```python
from build123d import *

# Parameters (mm, degrees)
F0_R     = 14.534071
F1_DEPTH = 4
F2_R     = 9.020601
F3_DEPTH = 55.9
F4_R     = 12.826106
F4_R_2   = 10.112728
F5_DEPTH = 67.3


with BuildPart() as f1:
    # F0 (on Top) → F1 (new body)
    with BuildSketch(Plane.XY):
        Circle(F0_R)
    extrude(amount=-F1_DEPTH)

    # F2 (on face) → F3 (join)
    with BuildSketch(Plane(origin=(0, 0, -4), x_dir=(1, 0, 0), z_dir=(0, 0, -1))):
        Circle(F2_R)
    extrude(amount=F3_DEPTH)

    # F4 (on face) → F5 (join)
    with BuildSketch(Plane(origin=(0, 0, -4), x_dir=(1, 0, 0), z_dir=(0, 0, -1))):
        Circle(F4_R)
        Circle(F4_R_2, mode=Mode.SUBTRACT)
    extrude(amount=F5_DEPTH)


solid = f1.part
```
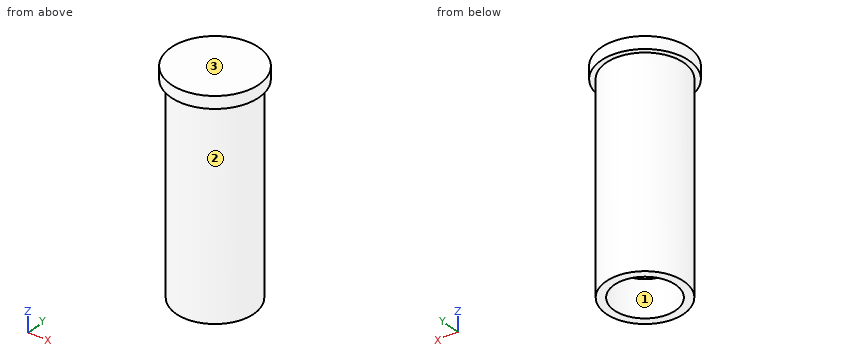
Geometry check sheet. Reference: the model listing, model coordinates, mm. Face numbers are marked on the shaded views. Give positions to 0.01 mm unless a question says otherwise; leave off trailing zeros. Order: outer loops, then holes, each group sorted by start corner. A loop starts at its lowest first (then second) coordinate and runs counter-clockwise, first axis right, second up. Notation, with made-up numbers: (6, 29.5) -> (48, 29.5) arc R20 ccw to (48, 44.5) -> close; hole circle Ø4 at (31.5, 37.25). An arc over 180 degrees is marked (long way). Write each question's results on one line, items separated by ' | '. Start each with the question number.
(1) Sectioned sample at B-B (x = 0). Enter the section's corners in (y, z), plus the area to 3 significant figures.
(2) Scan lines: line 1 (Y direction, x = 0, z = -51); line 2 (X direction, y = 0.5, z = -41); line 3 (Y direction, x = 3.5, z = -42). Record each from-to range of solid material in increasing order.
(3) Gauge pin test, flat ends, axial feed: P1, Ø10, axis at x = -1.5, y = 4.5, coming from the -Z side; P2, Ø5, axis at x = -8.5, z = -18.5, coming from the -Y side; P3, Ø1, axis at x = 1.5, z = -14.5, coming from the -Y side. Record the tip position at first contact, or that the pin passes through.
(4) Sectioned sample at A-A (z = -33). Enter the section's corners in (x, y), plus the area to 3 significant figures.
(5) Sectioned sample at D-D (y = 12). Enter the section's corners in (x, z).
(6) Mould release check, pull along Y, two halves, no side actions. Record for the marked faces 1, 2 and 3: pulls with the +Y half, pulls with the -Y half, needs draft (parallel to the pull), parting line crosses it, or undercut.
Answer below:
1) outline: (-14.53, -4) -> (-12.83, -4) -> (-12.83, -71.3) -> (-10.11, -71.3) -> (-10.11, -4) -> (-9.02, -4) -> (-9.02, -59.9) -> (9.02, -59.9) -> (9.02, -4) -> (10.11, -4) -> (10.11, -71.3) -> (12.83, -71.3) -> (12.83, -4) -> (14.53, -4) -> (14.53, 0) -> (-14.53, 0) -> close | area: 1,490 mm2
2) line 1: -12.83 to -10.11, -9.02 to 9.02, 10.11 to 12.83 | line 2: -12.82 to -10.1, -9.01 to 9.01, 10.1 to 12.82 | line 3: -12.34 to -9.49, -8.31 to 8.31, 9.49 to 12.34
3) P1: z = -59.9 | P2: y = -11.34 | P3: y = -12.79
4) outline: circle Ø25.65 at (0, 0); circle Ø18.04 at (0, 0); hole circle Ø20.23 at (0, 0) | area: 451 mm2
5) outline: (-8.2, -4) -> (-4.53, -4) -> (-4.53, -71.3) -> (4.53, -71.3) -> (4.53, -4) -> (8.2, -4) -> (8.2, 0) -> (-8.2, 0) -> close
6) face 1: undercut | face 2: parting line crosses it | face 3: needs draft
